```python
from build123d import *

# Parameters (mm, degrees)
PAD_DEPTH    = 1100
SKETCH001_R  = 6
POCKET_DEPTH = 80.001


with BuildPart() as part:
    # Sketch → Pad (new body)
    with BuildSketch(Plane.XY):
        with BuildLine():
            Line((0, 0), (0, 45))
            Line((0, 45), (80, 45))
            Line((80, 45), (80, 0))
            Line((80, 0), (78, 0))
            ThreePointArc((75.011416, 2.738533), (75.973229, 0.788168), (78, 0))
            Line((75.011416, 2.738533), (72.437925, 32.153668))
            ThreePointArc((72.437925, 32.153668), (70.033391, 37.02958), (64.966465, 39))
            Line((64.966465, 39), (15.033535, 39))
            ThreePointArc((15.033535, 39), (9.966609, 37.02958), (7.562075, 32.153668))
            Line((4.988584, 2.738533), (7.562075, 32.153668))
            ThreePointArc((2, 0), (4.026771, 0.788168), (4.988584, 2.738533))
            Line((0, 0), (2, 0))
        make_face()
    extrude(amount=PAD_DEPTH)

    # Sketch001 (on Face2 of Pad) → Pocket (cut, through all)
    with BuildSketch(Plane(origin=(0, 0, 0), x_dir=(0, -1, 0), z_dir=(-1, 0, 0))):
        with Locations((-62, 1050)):
            Circle(SKETCH001_R)
    extrude(amount=-POCKET_DEPTH, mode=Mode.SUBTRACT)


solid = part.part
```
Work out the finished part from the listing and answer in its coordinate system (mm). A direction names the side the tool comes from. Round coordinates to 2 decimals unless told otherwise and drop trailing zeros. Write each loop counter-clockwise with the first axis right and the second up, starting at its lowest first coordinate (ties: lowest second). Pieces come first, ordered by that corner, then holes. Notation, with made-up numbers: (33, -29) -> (47, -29) arc R18 cw to (47, -15) -> close; hole circle Ø4 at (13, 5). An arc over 180 degrees is marked (long way). Write each question's results on one line, items separated by ' | '.
1) For a pull along X with two mould halves and no side action, classify faces 1 (the flat face through (73.743, 17.24, 542.3)), 2 (the flat face through (0, 22, 542)), 3 (the flat face through (43.1, 39.3, 0)) as +X half, -X half, draft (parallel to the pull), parting line (faces both ways), or undercut.
Findings:
face 1: undercut | face 2: -X half | face 3: draft
2) The part is cut by section B-B (z = 493). Write down the section's boundary in (x, y).
Findings:
outline: (0, 0) -> (2, 0) arc R3 ccw to (4.99, 2.74) -> (7.56, 32.15) arc R7.5 cw to (15.03, 39) -> (64.97, 39) arc R7.5 cw to (72.44, 32.15) -> (75.01, 2.74) arc R3 ccw to (78, 0) -> (80, 0) -> (80, 45) -> (0, 45) -> close
3) The part is cut by section C-C (x = 26). Write down the section's boundary in (y, z), and give its area (3 significant figures).
Findings:
outline: (39, 0) -> (45, 0) -> (45, 1100) -> (39, 1100) -> close | area: 6,600 mm²
4) Consider line 1 along Y through (x, z) = (26.5, 506.5); line 2 along X through (y, z) = (2, 345); line 3 along X through (y, z) = (6.5, 579.5). Determine where each line is inside the solid, lowest interval first. Write a range as [from, to].
Findings:
line 1: y = [39, 45] | line 2: x = [0, 4.83], [75.17, 80] | line 3: x = [0, 5.32], [74.68, 80]
5) Which of the six approach directions +Z, -Z, +X, -X, +Y, -Y give full straight-line access (tool end or side, diameter ignored) to faces 4 (the flat face through (6.257, 17.24, 542.3)), 5 (the flat face through (39, 45, 542))?
Findings:
face 4: +Z, -Z, -Y | face 5: +Z, -Z, +X, -X, +Y
6) A flat-ended cylindrical pin translates along its axis: pin 1 (4 mm diameter, centred on y = 6.5, z = 226, fed in from -X). Find the tip coordinate at first contact, or state that the pin passes through.
Findings:
pin 1: stops at x = 0
7) The part is cut by section A-A (y = 15). Write down the section's boundary in (x, z).
Findings:
outline: (0, 0) -> (6.06, 0) -> (6.06, 1100) -> (0, 1100) -> close; (73.94, 0) -> (80, 0) -> (80, 1100) -> (73.94, 1100) -> close
